The model under review builds one solid part; all positions refer to its coordinate system, in mm. A direction names the side the tool comes from. Coordinates: 2 decimals unless noted, no trailing zeros. Loops run counter-clockwise (first coordinate to the right, second up) from the corner with the lowest first, then second, coordinate; pieces in that order, holes last. Notation, with made-up numbers: M 26,-33 L 36,-33 A27 cw 36,4 Z; hole C 74.25,77.25 d11. An arc over 180 degrees is marked long. Return JSON: item names as keys, results as strings.
```python
from build123d import *

# Parameters (mm, degrees)
SKETCH1_R               = 10
BOSS_EXTRUDE2_DEPTH     = 15
FILLET3_R               = 25
F_3DSKETCH1_R           = 10
BOSS_EXTRUDE5_DEPTH     = 16
FILLET5_R               = 16
BOSS_EXTRUDE6_START     = -72.295744394
BOSS_EXTRUDE6_OUTLINE_R = 25
BOSS_EXTRUDE6_DEPTH     = 42
SKETCH2_R               = 14
CUT_EXTRUDE1_DEPTH      = 56
CUT_EXTRUDE2_START      = -5
CUT_EXTRUDE2_DEPTH      = 5


# Read off the part's stored shape, not the designer's step: Boss-Extrude6
with BuildPart() as part:
    # Sketch1 → Boss-Extrude2 (new body)
    with BuildSketch(Plane(origin=(0, 0, 0), x_dir=(1, 0, 0), z_dir=(0, 1, 0))):
        Polygon((-60.127867878, 66.295744394), (81.872132122, 66.295744394), (81.872132122, -3.704255606), (-60.127867878, -23.704255606), align=None)
        with Locations(Location((-35.127867878, 1.295744394, 0), (0, 0, 270))):
            Circle(SKETCH1_R, mode=Mode.SUBTRACT)
        with Locations(Location((56.872132122, 26.295744394, 0), (0, 0, 270))):
            Circle(SKETCH1_R, mode=Mode.SUBTRACT)
    extrude(amount=BOSS_EXTRUDE2_DEPTH)

    # Fillet3
    fillet3_edges = [part.edges().sort_by_distance(p)[0] for p in [
        (81.872132122, 7.5, 3.704255606),
        (-60.127867878, 7.5, 23.704255606),
    ]]
    fillet(fillet3_edges, radius=FILLET3_R)

    # 3DSketch1 → Boss-Extrude5 (add)
    with BuildSketch(Plane(origin=(-60.127867878, 15, -66.295744394), x_dir=(1, 0, 0), z_dir=(0, 0, 1))):
        Polygon((0, 0), (142, 0), (105, 35), (50, 35), (50, 60), (0, 60), align=None)
        with Locations((97, 20)):
            Circle(F_3DSKETCH1_R, mode=Mode.SUBTRACT)
    extrude(amount=BOSS_EXTRUDE5_DEPTH)

    # Fillet5
    fillet5_edges = [part.edges().sort_by_distance(p)[0] for p in [
        (44.872132122, 50, -58.295744394),
    ]]
    fillet(fillet5_edges, radius=FILLET5_R)

    # Boss-Extrude6 outline → Boss-Extrude6 (add)
    with BuildSketch(Plane.XY.offset(BOSS_EXTRUDE6_START)):
        with Locations((-35.127867878, 75)):
            Circle(BOSS_EXTRUDE6_OUTLINE_R)
    extrude(amount=BOSS_EXTRUDE6_DEPTH)

    # Sketch2 → Cut-Extrude1 (cut)
    with BuildSketch(Plane.XY.offset(-30.295744394)):
        with Locations((-35.127867878, 75)):
            Circle(SKETCH2_R)
    extrude(amount=-CUT_EXTRUDE1_DEPTH, mode=Mode.SUBTRACT)

    # 3DSketch3 → Cut-Extrude2 (cut)
    with BuildSketch(Plane(origin=(-20.127867878, 95, -30.295744394), x_dir=(-0.5999999999999998, -0.8000000000000002, 0), z_dir=(0, 0, 1)).offset(CUT_EXTRUDE2_START)):
        with BuildLine():
            Line((0, 0), (32, 24))
            ThreePointArc((32, 24), (45, 15), (50, 0))
            Line((50, 0), (18, -24))
            ThreePointArc((18, -24), (5, -15), (0, 0))
        make_face()
    extrude(amount=CUT_EXTRUDE2_DEPTH, mode=Mode.SUBTRACT)


solid = part.part
```
1. To check wall thickness, follow line 1 (X direction, y = 74.5, z = -37.5); line 2 (Z direction, x = -12, y = 56.5); line 3 (Y direction, x = 49.5, z = -48.5). State the ranges of each line that lie inside material, in increasing order.
Check values:
{"line 1": "-60.12 to -49.12, -21.14 to -10.13", "line 2": "-66.3 to -50.3", "line 3": "0 to 15"}
2. Insertion check: pin 1 Ø5 at (x, z) = (24, -56) entering from +Y; pin 2 Ø4 at (y, z) = (52.5, -37) entering from -X; pin 3 Ø16 at (x, y) = (36.87, 35) entering from +Z; pin 4 Ø24 at (x, y) = (-29.5, 86.5) entering from +Z. Each pin has a flat end and moves straight along its axis. Give the tip position at first contact, or say it passes through.
Check values:
{"pin 1": "y = 50", "pin 2": "x = -49.44", "pin 3": "through", "pin 4": "z = -30.3"}
3. The part is to be moulded in two halves that separate along X. For faces 1 (the face through (41.49, 26.13, -58.41)), 2 (the face through (-24, 64, -72.296)), 3 (the face through (-60.128, 21, -57)), 4 (the face through (75.906, 7.605, -1.813)), say which applies: released by +X, released by -X, zero draft, split by the parting line, or undercut.
Check values:
{"face 1": "undercut", "face 2": "zero draft", "face 3": "released by -X", "face 4": "released by +X"}
4. Add section D-D on x = 15.5. Give the boundary of the cut face in (y, z), plus the area to 3 significant figures.
Check values:
{"outline": "M 0,-66.3 L 50,-66.3 L 50,-50.3 L 15,-50.3 L 15,13.05 L 0,13.05 Z", "area": "1,750 mm²"}
5. Add section B-B on y = 35. Give the boundary of the cut face in (x, z).
Check values:
{"outline": "M -60.13,-66.3 L 26.87,-66.3 L 26.87,-50.3 L -60.13,-50.3 Z; M 46.87,-66.3 L 60.73,-66.3 L 60.73,-50.3 L 46.87,-50.3 Z"}
6. Add section A-A on z = -42. Give the boundary of the cut face in (x, y).
Check values:
{"outline": "M -60.13,0 L 81.87,0 L 81.87,15 L -60.13,15 Z; C -35.13,75 d50; hole C -35.13,75 d28"}
7. Add section C-C on z = 3. Give the boundary of the cut face in (x, y).
Check values:
{"outline": "M -58.79,0 L -44.16,0 L -44.16,15 L -58.79,15 Z; M -26.1,0 L 70.4,0 L 70.4,15 L -26.1,15 Z"}
8. Machinability: for faces 5 (the face through (-21, 76, -35.296)), 6 (the face through (-44, 7.4, 3.32)), 7 (the face through (15, 50, -58)), 8 (the face through (15.003, 7.395, 13.122)), 9 (the face through (-16, 75, -30.296)), which of the approach directions +Z, -Z, +X, -X, +Y, -Y give a long, thin tool a straight path to every point of the face, cutting with its end or side? Answer none if there is none.
Check values:
{"face 5": "+Z, +Y", "face 6": "+Y, -Y", "face 7": "+Z, -Z, +X, +Y", "face 8": "+Z, +X, +Y, -Y", "face 9": "+Z, +X, -X, +Y"}
